from build123d import *

# Parameters (mm, degrees)
F0_W     = 31
F0_H     = 36
F1_DEPTH = 3.85
F2_SIZE2 = 5
F2_SIZE  = 5
F3_R     = 5
F5_DEPTH = 2.5
F6_SIZE  = 1


with BuildPart() as f1:
    # F0 (on Top) → F1 (new body)
    with BuildSketch(Plane.XY):
        with Locations((15.5, -18)):
            Rectangle(F0_W, F0_H)
    extrude(amount=F1_DEPTH)

    # F2
    f2_edges = [f1.edges().sort_by_distance(p)[0] for p in [
        (0, 0, 1.925),
    ]]
    chamfer(f2_edges, length=F2_SIZE, length2=F2_SIZE2)

    # F3
    f3_edges = [f1.edges().sort_by_distance(p)[0] for p in [
        (31, 0, 1.925),
        (31, -36, 1.925),
        (0, -36, 1.925),
    ]]
    fillet(f3_edges, radius=F3_R)

    # F4 (on face) → F5 (join)
    with BuildSketch(Plane.XY.offset(3.85)):
        with BuildLine():
            Line((5, -36), (6.05, -36))
            ThreePointArc((6.05, -36), (6.95, -35.7), (7.85, -36))
            Line((7.85, -36), (24.05, -36))
            ThreePointArc((24.05, -36), (24.95, -35.7), (25.85, -36))
            Line((25.85, -36), (26, -36))
            ThreePointArc((26, -36), (29.5355339059, -34.5355339059), (31, -31))
            Line((31, -31), (31, -5))
            ThreePointArc((31, -5), (29.5355339059, -1.4644660941), (26, 0))
            Line((26, 0), (5, 0))
            Line((5, 0), (0, -5))
            Line((0, -5), (0, -31))
            ThreePointArc((0, -31), (1.4644660941, -34.5355339059), (5, -36))
        make_face()
        with BuildLine():
            Line((23.45, -33.8), (8.45, -33.8))
            ThreePointArc((8.45, -33.8), (5.8893398282, -34.8606601718), (6.95, -32.3))
            Line((6.95, -32.3), (6.95, -8.2))
            ThreePointArc((6.95, -8.2), (5.8893398282, -5.6393398282), (8.45, -6.7))
            Line((8.45, -6.7), (23.45, -6.7))
            ThreePointArc((23.45, -6.7), (24.95, -5.2), (26.45, -6.7))
            ThreePointArc((26.45, -6.7), (26.0106601718, -7.7606601718), (24.95, -8.2))
            Line((24.95, -8.2), (24.95, -32.3))
            ThreePointArc((24.95, -32.3), (26.0106601718, -32.7393398282), (26.45, -33.8))
            ThreePointArc((26.45, -33.8), (24.95, -35.3), (23.45, -33.8))
        make_face(mode=Mode.SUBTRACT)
    extrude(amount=F5_DEPTH)

    # F6
    f6_edges = [f1.edges().sort_by_distance(p)[0] for p in [
        (6.95, -20.25, 6.35),
        (15.95, -6.7, 6.35),
        (24.95, -20.25, 6.35),
        (15.95, -33.8, 6.35),
    ]]
    chamfer(f6_edges, length=F6_SIZE)


solid = f1.part
Can you work these out from the model? Positions are in its coordinate system, mm. A direction names the side the tool comes from. Give positions to 0.01 mm unless a question says otherwise; leave off trailing zeros. Loops run counter-clockwise (first coordinate to the right, second up) from the corner with the lowest first, then second, coordinate; pieces in that order, holes last. Notation, with made-up numbers: (-14, -23.75) - (28, -23.75) arc R33 cw to (28, 15.25) - close; hole circle Ø10 at (39, -30.5). An arc over 180 degrees is marked (long way). Answer as a JSON object with one key per item and string values.
Q1. If I drill on L1, parallel to Y at x = 11, z = 5.25; L2, parallel to X at y = -6.7, z = 5.55; L3, parallel to Z at x = 12, y = -26.5, over which ranges is the centre line in solid material (lowest first)?
Geometry says:
{"L1": "-36 to -33.8, -6.7 to 0", "L2": "0 to 5.45, 26.45 to 31", "L3": "0 to 3.85"}
Q2. Imagine slicing it at B-B on y = -20.5. Write out the boundary of the cut face in (x, z).
Geometry says:
{"outline": "(0, 0) - (31, 0) - (31, 6.35) - (25.95, 6.35) - (24.95, 5.35) - (24.95, 3.85) - (6.95, 3.85) - (6.95, 5.35) - (5.95, 6.35) - (0, 6.35) - close"}
Q3. Which directions (+Z, -Z, +X, -X, +Y, -Y) give clear straight access to the entire face, cutting with the end or side of a thin tool? Please do faces 1 (the flat face through (15, -18, 0)), 2 (the flat face through (6.95, -20, 5)), 3 (the cylindrical face through (6.9, -35.7, 5.1)).
Geometry says:
{"face 1": "-Z, +X, -X, +Y, -Y", "face 2": "+Z", "face 3": "+Z, -Y"}
Q4. Will these pins go through, and if not, where does the flat tip stop? P1, Ø6, axis at x = 18.5, y = -21.5, coming from the +Z side; P2, Ø5, axis at x = 6.95, y = -33.8, coming from the +Z side.
Geometry says:
{"P1": "z = 3.85", "P2": "z = 6.35"}
Q5. Imagine slicing it at A-A on z = 3.25. Write out the boundary of the cut face in (x, y).
Geometry says:
{"outline": "(0, -31) arc R5 ccw to (5, -36) - (26, -36) arc R5 ccw to (31, -31) - (31, -5) arc R5 ccw to (26, 0) - (5, 0) - (0, -5) - close"}
Q6. Imagine slicing it at C-C on x = 11.5. Write out the boundary of the cut face in (y, z), plus the area to 3 significant figures.
Geometry says:
{"outline": "(-36, 0) - (0, 0) - (0, 6.35) - (-5.7, 6.35) - (-6.7, 5.35) - (-6.7, 3.85) - (-33.8, 3.85) - (-33.8, 5.35) - (-34.8, 6.35) - (-36, 6.35) - close", "area": "160 mm²"}
Q7. If we mould it in two halves opening along Y, with no side actions, what happens to faces 4 (the cylindrical face through (24.9, -35.7, 5.1)), 5 (the flat face through (3, -2, 3)), 6 (the flat face through (16.06, -34.29, 5.84))? For each: pulls with the +Y half, pulls with the -Y half, needs draft (parallel to the pull), parting line crosses it, or undercut.
Geometry says:
{"face 4": "pulls with the -Y half", "face 5": "pulls with the +Y half", "face 6": "undercut"}
